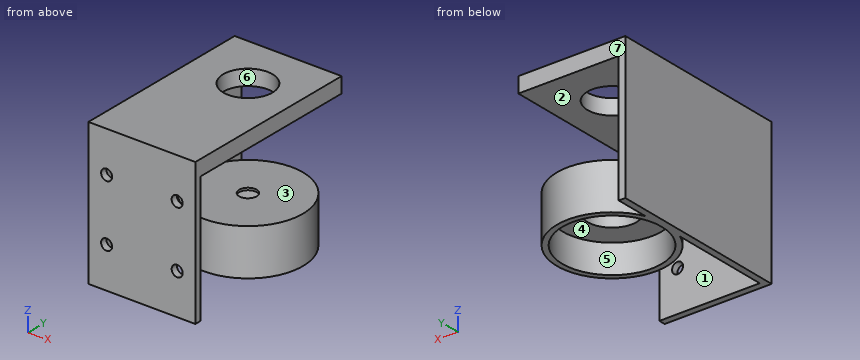
from build123d import *

# Parameters (mm, degrees)
SKETCH2_W           = 48.5
SKETCH2_H           = 65
SKETCH2_R           = 2.5
BOSS_EXTRUDE1_DEPTH = 3
BOSS_EXTRUDE2_DEPTH = 80
SKETCH6_R           = 22.5
BOSS_EXTRUDE3_DEPTH = 13
BOSS_EXTRUDE4_DEPTH = 8
SKETCH12_R          = 11.1
CUT_EXTRUDE1_DEPTH  = 7
SKETCH13_R          = 4
CUT_EXTRUDE2_DEPTH  = 78
SKETCH14_R          = 11.15
CUT_EXTRUDE3_DEPTH  = 10


with BuildPart() as part:
    # Sketch2 → Boss-Extrude1 (new body)
    with BuildSketch(Plane(origin=(0, 0, 0), x_dir=(1, 0, 0), z_dir=(0, 1, 0))):
        Rectangle(SKETCH2_W, SKETCH2_H)
        with Locations(Location((-16, 14, 0), (0, 0, 270))):
            Circle(SKETCH2_R, mode=Mode.SUBTRACT)
        with Locations(Location((16, 14, 0), (0, 0, 90))):
            Circle(SKETCH2_R, mode=Mode.SUBTRACT)
        with Locations(Location((16, -14, 0), (0, 0, 270))):
            Circle(SKETCH2_R, mode=Mode.SUBTRACT)
        with Locations(Location((-16, -14, 0), (0, 0, 90))):
            Circle(SKETCH2_R, mode=Mode.SUBTRACT)
    extrude(amount=BOSS_EXTRUDE1_DEPTH)

    # Sketch3 → Boss-Extrude2 (add)
    with BuildSketch(Plane(origin=(0, 3, 0), x_dir=(1, 0, 0), z_dir=(0, 1, 0))):
        Polygon((-24.25, 32.5), (-24.25, -32.5), (24.25, -32.5), (24.25, -25.5), (-21.25, -25.5), (-21.25, 32.5), align=None)
    extrude(amount=BOSS_EXTRUDE2_DEPTH)

    # Sketch6 → Boss-Extrude3 (add)
    with BuildSketch(Plane(origin=(0, 0, -32.5), x_dir=(-1, 0, 0), z_dir=(0, 0, -1))):
        with BuildLine():
            Line((21.25, 67.797958971), (21.25, 48.202041029))
            ThreePointArc((21.25, 48.202041029), (-26.75, 58), (21.25, 67.797958971))
        make_face()
        with Locations((-1.75, 58)):
            Circle(SKETCH6_R, mode=Mode.SUBTRACT)
    extrude(amount=-BOSS_EXTRUDE3_DEPTH)

    # Sketch10 → Boss-Extrude4 (add)
    with BuildSketch(Plane.XY.offset(-19.5)):
        with BuildLine():
            Line((-21.25, 67.797958971), (-21.25, 48.202041029))
            ThreePointArc((-21.25, 48.202041029), (26.75, 58), (-21.25, 67.797958971))
        make_face()
    extrude(amount=BOSS_EXTRUDE4_DEPTH)

    # Sketch12 → Cut-Extrude1 (cut)
    with BuildSketch(Plane(origin=(0, 0, -19.5), x_dir=(-1, 0, 0), z_dir=(0, 0, -1))):
        with Locations((-1.75, 58)):
            Circle(SKETCH12_R)
    extrude(amount=-CUT_EXTRUDE1_DEPTH, mode=Mode.SUBTRACT)

    # Sketch13 → Cut-Extrude2 (cut)
    with BuildSketch(Plane(origin=(0, 0, -12.5), x_dir=(-1, 0, 0), z_dir=(0, 0, -1))):
        with Locations((-1.75, 58)):
            Circle(SKETCH13_R)
    extrude(amount=-CUT_EXTRUDE2_DEPTH, mode=Mode.SUBTRACT)

    # Sketch14 → Cut-Extrude3 (cut)
    with BuildSketch(Plane(origin=(0, 0, 25.5), x_dir=(-1, 0, 0), z_dir=(0, 0, -1))):
        with Locations((-1.75, 58)):
            Circle(SKETCH14_R)
    extrude(amount=-CUT_EXTRUDE3_DEPTH, mode=Mode.SUBTRACT)


solid = part.part
Design review of the part built by this model. Coordinates are the model's own, in mm. Face numbers are marked on the shaded views. A direction names the side the tool comes from. Give positions to 0.01 mm unless a question says otherwise; leave off trailing zeros. Order: outer loops, then holes, each group sorted by start corner. A loop starts at its lowest first (then second) coordinate and runs counter-clockwise, first axis right, second up.
1. Tool access review of the marked faces 5, 6 and 7: name each direction out of +Z, -Z, +X, -X, +Y, -Y from which nothing blocks a thin tool from reaching the whole face with its end or side.
Solution:
face 5: -Z
face 6: +Z
face 7: +Z, -Z, +X, -X, +Y
2. Add section D-D, the plane z = -14. State the section outline as (x, y) points.
Solution:
outline: (-24.25, 0) - (-18.5, 0) - (-18.5, 3) - (-21.25, 3) - (-21.25, 48.2) arc R25 ccw (long way) to (-21.25, 67.8) - (-21.25, 83) - (-24.25, 83) - close; (-13.5, 0) - (13.5, 0) - (13.5, 3) - (-13.5, 3) - close; (18.5, 0) - (24.25, 0) - (24.25, 3) - (18.5, 3) - close; hole circle Ø22.2 at (1.75, 58)
3. Add section C-C, the plane z = 14. State the section outline as (x, y) points.
Solution:
outline: (-24.25, 0) - (-18.5, 0) - (-18.5, 3) - (-21.25, 3) - (-21.25, 83) - (-24.25, 83) - close; (-13.5, 0) - (13.5, 0) - (13.5, 3) - (-13.5, 3) - close; (18.5, 0) - (24.25, 0) - (24.25, 3) - (18.5, 3) - close
4. Add section B-B, the plane x = 1.75. State the section outline as (y, z) points.
Solution:
outline: (0, -32.5) - (3, -32.5) - (3, 25.5) - (46.85, 25.5) - (46.85, 32.5) - (0, 32.5) - close; (33, -32.5) - (35.5, -32.5) - (35.5, -19.5) - (46.9, -19.5) - (46.9, -12.5) - (54, -12.5) - (54, -11.5) - (33, -11.5) - close; (62, -12.5) - (69.1, -12.5) - (69.1, -19.5) - (80.5, -19.5) - (80.5, -32.5) - (83, -32.5) - (83, -11.5) - (62, -11.5) - close; (69.15, 25.5) - (83, 25.5) - (83, 32.5) - (69.15, 32.5) - close
5. To check wall thickness, follow L1, parallel to X at y = 1.7, z = -14; L2, parallel to Z at x = 9, y = 69; L3, parallel to X at y = 73.5, z = -27. State the ranges of each line that lie inside material, in increasing order.
Solution:
L1: x = -24.25 to -18.5, -13.5 to 13.5, 18.5 to 24.25
L2: z = -19.5 to -11.5, 25.5 to 32.5
L3: x = -24.25 to -21.25, -17.87 to -14.56, 18.06 to 21.37
6. Add section A-A, the plane y = 58. State the section outline as (x, z) points, then the cut area to 3 significant figures.
Solution:
outline: (-24.25, -32.5) - (-20.75, -32.5) - (-20.75, -19.5) - (-9.35, -19.5) - (-9.35, -12.5) - (-2.25, -12.5) - (-2.25, -11.5) - (-21.25, -11.5) - (-21.25, 25.5) - (-9.4, 25.5) - (-9.4, 32.5) - (-24.25, 32.5) - close; (5.75, -12.5) - (12.85, -12.5) - (12.85, -19.5) - (24.25, -19.5) - (24.25, -32.5) - (26.75, -32.5) - (26.75, -11.5) - (5.75, -11.5) - close; (12.9, 25.5) - (24.25, 25.5) - (24.25, 32.5) - (12.9, 32.5) - close
area: 617 mm2
7. For pin 1 Ø13.5 at (x, y) = (1.75, 58) entering from +Z; pin 2 Ø8 at (x, z) = (-16, -14) entering from +Y; pin 3 Ø7 at (x, y) = (1.75, 58) entering from +Z; pin 4 Ø13.5 at (x, y) = (-3.5, 61) entering from -Z, all flat-tipped, find the tip position at first contact; note any pin that passes through.
Solution:
pin 1: stops at z = -11.5
pin 2: stops at y = 78.88
pin 3: passes through
pin 4: stops at z = -19.5
8. Mouldability with a two-part tool opening along Z and no side actions: class the marked faces 1, 2, 3 and 4 as +Z half, -Z half, draft (parallel to the pull), parting line (faces both ways), or undercut.
Solution:
face 1: draft
face 2: undercut
face 3: undercut
face 4: -Z half
